For this review, use the dimensioned drawing (mm, ordinates from the lowest corner) and the shaded views. A direction names the side the tool comes from. Coordinates: 2 decimals unless noted, no trailing zeros. Write each loop counter-clockwise with the first axis right and the second up, starting at its lowest first coordinate (ties: lowest second). Pieces come first, ordered by that corner, then holes. Notation, with made-up numbers: (77, 77) -> (128, 77) arc R8 ccw to (128, 83) -> close; hole circle Ø5 at (59, -17). An arc over 180 degrees is marked (long way). Return JSON: item names as keys, results as strings. Group by question number.
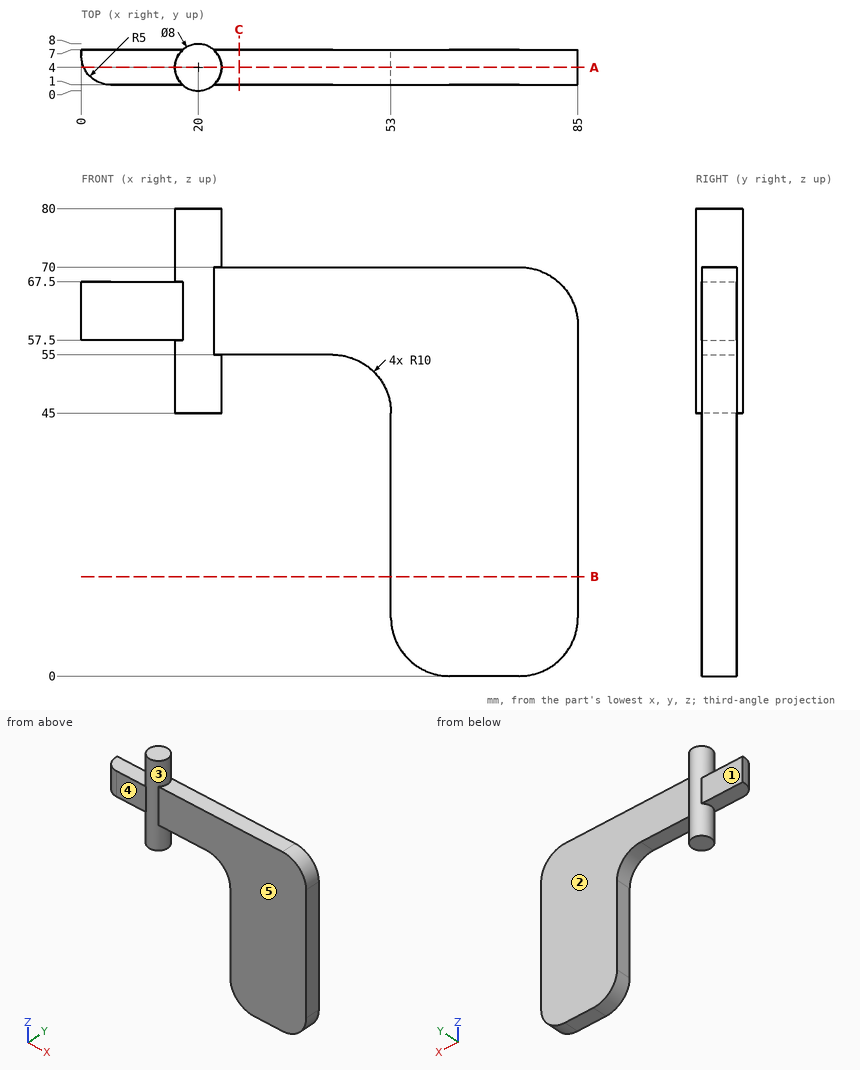
Q1. We need section C-C on x = 27. Write out the cut boundary in (y, z).
Q2. Wall thickness on L1, parallel to X at y = 3.75, z = 29; L2, parallel to X at y = 1.25, z = 54; L3, parallel to Z at x = 73.5, y = 4.25: over which ranges is each line inside the solid? List them lowest first.
Q3. For P1, Ø6, axis at x = 66.5, z = 62.5, coming from the +Y side; P2, Ø12, axis at x = 20.5, z = 65, coming from the +Y side; P3, Ø3, axis at x = 8, z = 64.5, coming from the -Y side; P4, Ø1.8, axis at x = 6, y = 5, coming from the -Z side, all flat-tipped, find the tip position at first contact; note any pin that passes through.
Q4. For the marked faces 1, 2, 3, 4 and 5, list the 3-axis set-ups (+Z, -Z, +X, -X, +Y, -Y) from which the entire face can be reached by the end or side of a thin tool; tool diameter is ignored.
Q5. We need section A-A on y = 4. Write out the cut boundary in (x, z).
Q6. We need section B-B on z = 17. Write out the cut boundary in (x, y).
Findings below:
{
 "1": {"outline": "(1, 55) -> (7, 55) -> (7, 70) -> (1, 70) -> close"},
 "2": {"L1": "x = 53 to 85", "L2": "x = 17.1 to 22.9, 47.36 to 85", "L3": "z = 0 to 70"},
 "3": {"P1": "stops at y = 7", "P2": "stops at y = 8", "P3": "stops at y = 1", "P4": "stops at z = 57.5"},
 "4": {"face 1": "+Z, -Z, -X, +Y", "face 2": "+Z, -Z, +X, +Y", "face 3": "none", "face 4": "+Z, -Z, -X, -Y", "face 5": "+Z, -Z, +X, -Y"},
 "5": {"outline": "(0.42, 57.5) -> (16, 57.5) -> (16, 45) -> (24, 45) -> (24, 55) -> (43, 55) arc R10 cw to (53, 45) -> (53, 10) arc R10 ccw to (63, 0) -> (75, 0) arc R10 ccw to (85, 10) -> (85, 60) arc R10 ccw to (75, 70) -> (24, 70) -> (24, 80) -> (16, 80) -> (16, 67.5) -> (0.42, 67.5) -> close"},
 "6": {"outline": "(53, 1) -> (85, 1) -> (85, 7) -> (53, 7) -> close"}
}
